from build123d import *

# Parameters (mm, degrees)
SKETCH_1_W          = 5
SKETCH_1_H          = 5
EXTRUDE_1_DEPTH     = 51
SKETCH_2_R          = 1.5
CUT_EXTRUDE_1_DEPTH = 52.122402134
SKETCH_3_W          = 3
SKETCH_3_H          = 5
EXTRUDE_2_DEPTH     = 7
FILLET_1_R          = 2.5
SKETCH_4_R          = 1.5
CUT_EXTRUDE_2_DEPTH = 59.268773799
SKETCH_5_W          = 3
SKETCH_5_H          = 5
EXTRUDE_3_DEPTH     = 7
FILLET_2_R          = 2.5
SKETCH_6_R          = 1.5
CUT_EXTRUDE_3_DEPTH = 59.131316861
FILLET_3_R          = 0.8


with BuildPart() as part:
    # 草图1 → 凸台-拉伸1 (new body)
    with BuildSketch(Plane.XY):
        Rectangle(SKETCH_1_W, SKETCH_1_H)
    extrude(amount=EXTRUDE_1_DEPTH)

    # 草图2 → 切除-拉伸1 (cut, through all)
    with BuildSketch(Plane.XY.offset(51)):
        Circle(SKETCH_2_R)
    extrude(amount=-CUT_EXTRUDE_1_DEPTH, mode=Mode.SUBTRACT)

    # 草图3 → 凸台-拉伸2 (add)
    with BuildSketch(Plane.XY.offset(51)):
        with Locations((-1, 0)):
            Rectangle(SKETCH_3_W, SKETCH_3_H)
    extrude(amount=EXTRUDE_2_DEPTH)

    # 圆角1
    fillet_1_edges = [part.edges().sort_by_distance(p)[0] for p in [
        (-1, -2.5, 58),
        (-1, 2.5, 58),
    ]]
    fillet(fillet_1_edges, radius=FILLET_1_R - 0.0001)  # a hair under: the kernel refuses the full size

    # 草图4 → 切除-拉伸2 (cut, through all)
    with BuildSketch(Plane.ZY.offset(2.5)):
        with Locations(Location((54.5, 0, 0), (0, 0, 270))):
            Circle(SKETCH_4_R)
    extrude(amount=-CUT_EXTRUDE_2_DEPTH, mode=Mode.SUBTRACT)

    # 草图5 → 凸台-拉伸3 (add)
    with BuildSketch(Plane(origin=(0, 0, 0), x_dir=(-1, 0, 0), z_dir=(0, 0, -1))):
        with Locations((1, 0)):
            Rectangle(SKETCH_5_W, SKETCH_5_H)
    extrude(amount=EXTRUDE_3_DEPTH)

    # 圆角2
    fillet_2_edges = [part.edges().sort_by_distance(p)[0] for p in [
        (-1, -2.5, -7),
        (-1, 2.5, -7),
    ]]
    fillet(fillet_2_edges, radius=FILLET_2_R - 0.0001)  # a hair under: the kernel refuses the full size

    # 草图6 → 切除-拉伸3 (cut, through all)
    with BuildSketch(Plane(origin=(0.5, 0, 0), x_dir=(0, 0, -1), z_dir=(1, 0, 0))):
        with Locations((3.5, 0)):
            Circle(SKETCH_6_R)
    extrude(amount=-CUT_EXTRUDE_3_DEPTH, mode=Mode.SUBTRACT)

    # 圆角3
    fillet_3_edges = [part.edges().sort_by_distance(p)[0] for p in [
        (-2.5, 1.767796242, 57.267796242),
        (-2.5, -1.767796242, 57.267796242),
        (-2.5, -2.5, 25.5),
        (-2.5, -1.767796242, -6.267796242),
        (-2.5, 1.767796242, -6.267796242),
        (-2.5, 2.5, 25.5),
        (2.5, -2.5, 25.5),
        (2.5, 2.5, 25.5),
    ]]
    fillet(fillet_3_edges, radius=FILLET_3_R)


solid = part.part
Work out the finished part from the listing and answer in its coordinate system (mm). A direction names the side the tool comes from. Give positions to 0.01 mm unless a question says otherwise; leave off trailing zeros. Loops run counter-clockwise (first coordinate to the right, second up) from the corner with the lowest first, then second, coordinate; pieces in that order, holes last. Notation, with made-up numbers: (47, 53.25) - (61, 53.25) arc R9 cw to (61, 61.25) - close; hole circle Ø5 at (89, -29). An arc over 180 degrees is marked (long way). Answer in a Markdown table with one row per item. Add a question column.
Q1. Each of these flat-tipped pins is pushed along its axis until it touches: P1, Ø2, axis at x = -0.5, y = 0.5, coming from the -Z side; P2, Ø1, axis at x = 1.5, y = -1, coming from the +Z side; P3, Ø2.5, axis at y = 0.5, z = 54.5, coming from the +X side. Where does it stop, or does it pass through?
Q2. The part is cut by section C-C (x = -0.8). State how many separate pieces and enclosed holes the cut face has, and give its area (3 significant figures).
Q3. A tool of negligible diameter and unlimited length cuts with its end or side. For faces 5 (the flat face through (0.5, 1, -2)), 6 (the flat face through (2, 0, 51)), 7 (the flat face through (2.5, 0, 25)), 8 (the cylindrical face through (-1.5, 0.07, 25.86)), from which of +Z, -Z, +X, -X, +Y, -Y can it reach the whole face along a straight path? Write none if from no direction.
Q4. Determine the mould class of faces 1 (the flat face through (2, 0, 0)), 2 (the flat face through (0, 0, 51)), 3 (the cylindrical face through (-1, 0, 53)), 4 (the flat face through (0, -2.5, 26)) for opening direction Z: released by +Z, released by -Z, zero draft, split by the parting line, or undercut.
Q5. The part is cut by section A-A (z = 14). Determine the outline of the cut face in (x, y), and give its area (3 significant figures).
Q6. Consider line 1 along Z through (x, y) = (-0.95, 0.05); line 2 along Y through (x, z) = (-1.6, -3.5); line 3 along Z through (x, y) = (-2.3, -0.65). Determine where each line is inside the solid, lowest interval first.
Q7. The part is cut by section B-B (z = 54.5). Determine the outline of the cut face in (x, y).
Solution:
| question | item | result |
|---|---|---|
| 1 | P1 | stops at z = -7 |
| 1 | P2 | stops at z = 51 |
| 1 | P3 | stops at x = 0.5 |
| 2 | separate pieces | 1 |
| 2 | enclosed holes | 3 |
| 2 | area | 176 mm² |
| 3 | face 5 | -Z, +X, +Y, -Y |
| 3 | face 6 | +Z, +X, +Y, -Y |
| 3 | face 7 | +Z, -Z, +X, +Y, -Y |
| 3 | face 8 | none |
| 4 | face 1 | released by -Z |
| 4 | face 2 | undercut |
| 4 | face 3 | undercut |
| 4 | face 4 | zero draft |
| 5 | outline | (-2.5, -1.7) arc R0.8 ccw to (-1.7, -2.5) - (1.7, -2.5) arc R0.8 ccw to (2.5, -1.7) - (2.5, 1.7) arc R0.8 ccw to (1.7, 2.5) - (-1.7, 2.5) arc R0.8 ccw to (-2.5, 1.7) - close; hole circle Ø3 at (0, 0) |
| 5 | area | 17.4 mm² |
| 6 | line 1 | z = -7 to -5, -2 to 0, 51 to 53, 56 to 58 |
| 6 | line 2 | y = -2.5 to -1.5, 1.5 to 2.5 |
| 6 | line 3 | z = -6.63 to -4.85, -2.15 to 53.15, 55.85 to 57.63 |
| 7 | outline | (-2.5, -1.7) arc R0.8 ccw to (-1.7, -2.5) - (0.5, -2.5) - (0.5, -1.5) - (-2.5, -1.5) - close; (-2.5, 1.5) - (0.5, 1.5) - (0.5, 2.5) - (-1.7, 2.5) arc R0.8 ccw to (-2.5, 1.7) - close |
